from build123d import *

# Parameters (mm, degrees)
BASE_EXT_DEPTH            = 30
BASE_EXT_DEPTH_BACK       = 25
ESQUISSE1_W               = 165
ESQUISSE1_H               = 165
ESQUISSE1_R               = 2
ESQUISSE2_W               = 165
ESQUISSE2_H               = 165
ESQUISSE2_R               = 5
BASE_BAS_DEPTH            = 5
ACCES_START               = -6
ESQUISSE4_R               = 30
ACCES_ROUES_DEPTH         = 16
ESQUISSE7_R               = 2
VIDE_SUPPORT_MOTEUR_DEPTH = 5
ESQUISSE9_R               = 5
VIS_MOTEUR_10MM_DEPTH     = 2
ESQUISSE10_R              = 2
VIS_PATIN_DEPTH           = 5
VIDE_CROIX_DEPTH          = 11
VIDE_GUIDAGE_REACH        = 123.846


with BuildPart() as part:
    # Esquisse1 → BASE EXT (new, two sides: drawn at the far end of the back side and taken through both)
    with BuildSketch(Plane(origin=(0, 0, 0), x_dir=(1, 0, 0), z_dir=(0, 1, 0)).offset(-BASE_EXT_DEPTH_BACK)):
        Rectangle(ESQUISSE1_W, ESQUISSE1_H)
        with Locations(Location((-76.5, -76.5, 0), (0, 0, 270))):
            Circle(ESQUISSE1_R, mode=Mode.SUBTRACT)
        with Locations(Location((-76.5, 0, 0), (0, 0, 270))):
            Circle(ESQUISSE1_R, mode=Mode.SUBTRACT)
        with Locations(Location((76.5, -76.5, 0), (0, 0, 270))):
            Circle(ESQUISSE1_R, mode=Mode.SUBTRACT)
        with BuildLine():
            ThreePointArc((77.5, -69.066965626), (71.196699141, -71.196699141), (69.066965626, -77.5))
            Line((69.066965626, -77.5), (-69.066965626, -77.5))
            ThreePointArc((-69.066965626, -77.5), (-71.196699141, -71.196699141), (-77.5, -69.066965626))
            Line((-77.5, -69.066965626), (-77.5, -7.433034374))
            ThreePointArc((-77.5, -7.433034374), (-72.588712088, -6.399361443), (-69.428932188, -2.5))
            Line((-69.428932188, -2.5), (-7.071067812, -2.5))
            ThreePointArc((-7.071067812, -2.5), (0, -7.5), (7.071067812, -2.5))
            Line((7.071067812, -2.5), (69.428932188, -2.5))
            ThreePointArc((69.428932188, -2.5), (72.588712088, -6.399361443), (77.5, -7.433034374))
            Line((77.5, -7.433034374), (77.5, -69.066965626))
        make_face(mode=Mode.SUBTRACT)
        with Locations(Location((76.5, 0, 0), (0, 0, 270))):
            Circle(ESQUISSE1_R, mode=Mode.SUBTRACT)
        with BuildLine():
            Line((-7.071067812, 2.5), (-69.428932188, 2.5))
            ThreePointArc((-69.428932188, 2.5), (-72.588712088, 6.399361443), (-77.5, 7.433034374))
            Line((-77.5, 7.433034374), (-77.5, 69.066965626))
            ThreePointArc((-77.5, 69.066965626), (-71.196699141, 71.196699141), (-69.066965626, 77.5))
            Line((-69.066965626, 77.5), (-2, 77.5))
            Line((-2, 77.5), (-2, 7.228416147))
            ThreePointArc((-2, 7.228416147), (-5.114738276, 5.485385344), (-7.071067812, 2.5))
        make_face(mode=Mode.SUBTRACT)
        with Locations(Location((-76.5, 76.5, 0), (0, 0, 270))):
            Circle(ESQUISSE1_R, mode=Mode.SUBTRACT)
        with Locations(Location((0, 0, 0), (0, 0, 270))):
            Circle(ESQUISSE1_R, mode=Mode.SUBTRACT)
        with BuildLine():
            ThreePointArc((77.5, 7.433034374), (72.709235004, 6.471483659), (69.52750715, 2.76303157))
            Line((69.52750715, 2.76303157), (7.071067812, 2.5))
            ThreePointArc((7.071067812, 2.5), (5.114738276, 5.485385344), (2, 7.228416147))
            Line((2, 7.228416147), (2, 77.5))
            Line((2, 77.5), (69.066965626, 77.5))
            ThreePointArc((69.066965626, 77.5), (71.196699141, 71.196699141), (77.5, 69.066965626))
            Line((77.5, 69.066965626), (77.5, 7.433034374))
        make_face(mode=Mode.SUBTRACT)
        with Locations(Location((76.5, 76.5, 0), (0, 0, 270))):
            Circle(ESQUISSE1_R, mode=Mode.SUBTRACT)
    extrude(amount=BASE_EXT_DEPTH + BASE_EXT_DEPTH_BACK)

    # Esquisse2 → BASE BAS (add)
    with BuildSketch(Plane.XZ.offset(25)):
        Rectangle(ESQUISSE2_W, ESQUISSE2_H)
        with Locations(Location((-76.5, 0, 0), (0, 0, 270))):
            Circle(ESQUISSE2_R, mode=Mode.SUBTRACT)
        with Locations(Location((-76.5, -76.5, 0), (0, 0, 270))):
            Circle(ESQUISSE2_R, mode=Mode.SUBTRACT)
        with Locations(Location((76.5, -76.5, 0), (0, 0, 90))):
            Circle(ESQUISSE2_R, mode=Mode.SUBTRACT)
        with Locations(Location((76.5, 0, 0), (0, 0, 90))):
            Circle(ESQUISSE2_R, mode=Mode.SUBTRACT)
        with Locations(Location((76.5, 76.5, 0), (0, 0, 90))):
            Circle(ESQUISSE2_R, mode=Mode.SUBTRACT)
        with Locations(Location((0, 0, 0), (0, 0, 270))):
            Circle(ESQUISSE2_R, mode=Mode.SUBTRACT)
        with Locations(Location((-76.5, 76.5, 0), (0, 0, 270))):
            Circle(ESQUISSE2_R, mode=Mode.SUBTRACT)
    extrude(amount=BASE_BAS_DEPTH)

    # Esquisse4 → ACCES ROUES (cut)
    with BuildSketch(Plane(origin=(-77.5, 0, 0), x_dir=(0, 0, -1), z_dir=(1, 0, 0)).offset(ACCES_START)):
        with Locations((-38.25, -5.128631201)):
            Circle(ESQUISSE4_R)
    acces_roues = extrude(amount=ACCES_ROUES_DEPTH, mode=Mode.SUBTRACT)

    # SYM ACCES ROUE: ACCES ROUES across plane
    add(acces_roues.mirror(Plane(origin=(0, 0, 0), x_dir=(0, 0, 1), z_dir=(1, 0, 0))), mode=Mode.SUBTRACT)

    # Esquisse7 → VIDE SUPPORT MOTEUR (cut)
    with BuildSketch(Plane(origin=(0, -25, 0), x_dir=(1, 0, 0), z_dir=(0, 1, 0))):
        with Locations(Location((54.232363064, -61.25, 0), (0, 0, 270))):
            Circle(ESQUISSE7_R)
        with Locations(Location((31.732363064, -60.75, 0), (0, 0, 270))):
            Circle(ESQUISSE7_R)
        with Locations(Location((31.732363064, -15.75, 0), (0, 0, 270))):
            Circle(ESQUISSE7_R)
        with Locations(Location((54.232363064, -15.25, 0), (0, 0, 270))):
            Circle(ESQUISSE7_R)
        with Locations(Location((-54.232363064, -15.25, 0), (0, 0, 270))):
            Circle(ESQUISSE7_R)
        with Locations(Location((-31.732363064, -15.75, 0), (0, 0, 270))):
            Circle(ESQUISSE7_R)
        with Locations(Location((-31.732363064, -60.75, 0), (0, 0, 270))):
            Circle(ESQUISSE7_R)
        with Locations(Location((-54.232363064, -61.25, 0), (0, 0, 270))):
            Circle(ESQUISSE7_R)
    extrude(amount=-VIDE_SUPPORT_MOTEUR_DEPTH, mode=Mode.SUBTRACT)

    # Esquisse9 → VIS MOTEUR 10mm (cut)
    with BuildSketch(Plane.XZ.offset(30)):
        with Locations(Location((-54.232363064, 61.25, 0), (0, 0, 270))):
            Circle(ESQUISSE9_R)
        with Locations(Location((-31.732363064, 60.75, 0), (0, 0, 270))):
            Circle(ESQUISSE9_R)
        with Locations(Location((-54.232363064, 15.25, 0), (0, 0, 270))):
            Circle(ESQUISSE9_R)
        with Locations(Location((-31.732363064, 15.75, 0), (0, 0, 270))):
            Circle(ESQUISSE9_R)
        with Locations(Location((31.732363064, 15.75, 0), (0, 0, 90))):
            Circle(ESQUISSE9_R)
        with Locations(Location((54.232363064, 15.25, 0), (0, 0, 90))):
            Circle(ESQUISSE9_R)
        with Locations(Location((31.732363064, 60.75, 0), (0, 0, 90))):
            Circle(ESQUISSE9_R)
        with Locations(Location((54.232363064, 61.25, 0), (0, 0, 90))):
            Circle(ESQUISSE9_R)
    extrude(amount=-VIS_MOTEUR_10MM_DEPTH, mode=Mode.SUBTRACT)

    # Esquisse10 → VIS PATIN (cut)
    with BuildSketch(Plane.XZ.offset(30)):
        with Locations(Location((-42.5, -52.5, 0), (0, 0, 270))):
            Circle(ESQUISSE10_R)
        with Locations(Location((42.5, -52.5, 0), (0, 0, 270))):
            Circle(ESQUISSE10_R)
    extrude(amount=-VIS_PATIN_DEPTH, mode=Mode.SUBTRACT)

    # Esquisse11 → VIDE CROIX (cut)
    with BuildSketch(Plane.XY.offset(2.5)):
        Polygon((-69.428932188, 27.333215955), (-41.273544688, 2.5), (-69.428932188, -22.333215955), align=None)
        Polygon((-66.4053875, 30), (-38.25, 5.166784045), (-10.0946125, 30), align=None)
        Polygon((-7.071067812, -22.333215955), (-7.071067812, 27.333215955), (-35.226455312, 2.5), align=None)
        Polygon((-10.0946125, -25), (-66.4053875, -25), (-38.25, -0.166784045), align=None)
        Polygon((66.4053875, -25), (38.25, -0.166784045), (10.0946125, -25), align=None)
        Polygon((7.071067812, 27.333215955), (35.226455312, 2.5), (7.071067812, -22.333215955), align=None)
        Polygon((69.428932188, -22.333215955), (69.428932188, 27.333215955), (41.273544688, 2.5), align=None)
        Polygon((10.0946125, 30), (66.4053875, 30), (38.25, 5.166784045), align=None)
    extrude(amount=-VIDE_CROIX_DEPTH, mode=Mode.SUBTRACT)

    # VIDE GUIDAGE: up to this face of the body (flat: up to its plane)
    vide_guidage_end = Plane(part.part.faces().sort_by_distance((2, 2.5, -42.364208074))[0])
    # Esquisse12 → VIDE GUIDAGE (cut, up to the picked face)
    with BuildSketch(Plane.ZY.offset(2), mode=Mode.PRIVATE) as vide_guidage_sk1:
        Polygon((-7.228416147, 10), (-12.228416147, 10), (-12.228416147, 30), (-72.5, 30), (-72.5, 10), (-77.5, 10), (-77.5, -25), (-7.228416147, -25), align=None)
    vide_guidage_tool1 = split(extrude(vide_guidage_sk1.sketch, amount=-VIDE_GUIDAGE_REACH, mode=Mode.PRIVATE), bisect_by=vide_guidage_end, keep=Keep.BOTH, mode=Mode.PRIVATE)
    add(vide_guidage_tool1.solids().sort_by(Axis((-2, 1.545004, -42.364208), (1, 0, 0)))[0], mode=Mode.SUBTRACT)


solid = part.part
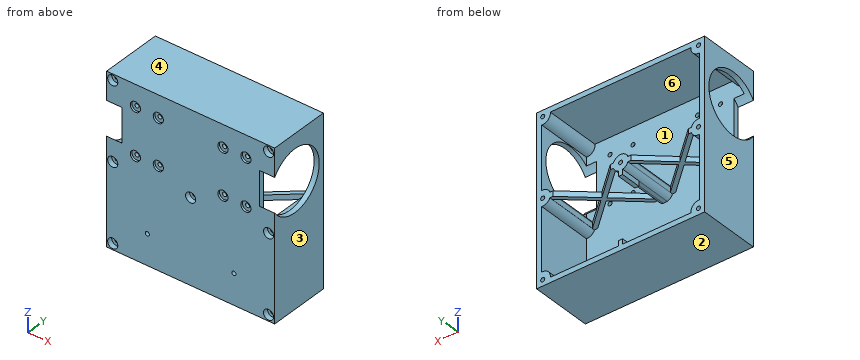
Input: part model. Units: mm. Frame: model coordinates. Face numbers are marked on the shaded views. A direction names the side the tool comes from. Give positions to 0.01 mm unless a question says otherwise; leave off trailing zeros. Order: outer loops, then holes, each group sorted by start corner. A loop starts at its lowest first (then second) coordinate and runs counter-clockwise, first axis right, second up. Notation, with made-up numbers: M 63.25,48.25 L 99.25,48.25 A3 ccw 99.25,53.25 Z; hole C 52,51 d1. An arc over 180 degrees is marked long. Answer as a JSON object with one key per item and string values.
1. Reachability of the marked faces 5 and 6 from +Z, -Z, +X, -X, +Y, -Y: full face, straight path, thin tool, end or side. Return the list, or none.
Result sheet:
{"face 5": "+Z, -Z, -X, +Y, -Y", "face 6": "+Y"}
2. Cut plane A-A, the plane z = 0. State how many separate pieces and enclosed holes the cut face has, and give its area (3 significant figures).
Result sheet:
{"separate pieces": "4", "enclosed holes": "6", "area": "3,500 mm²"}
3. Cut plane C-C, the plane z = -26. Output: boundary loops of the cut face in (x, y), and give its area (4 significant figures).
Result sheet:
{"outline": "M -82.5,-30 L 82.5,-30 L 82.5,30 L 77.5,30 L 77.5,-25 L -77.5,-25 L -77.5,30 L -82.5,30 Z", "area": "1,375 mm²"}
4. Cut plane B-B, the plane x = -24.5. Output: boundary loops of the cut face in (y, z).
Result sheet:
{"outline": "M -30,-82.5 L 30,-82.5 L 30,-77.5 L -25,-77.5 L -25,77.5 L 30,77.5 L 30,82.5 L -30,82.5 Z; M -12.29,-2.5 L -6.96,-2.5 L -6.96,2.5 L -12.29,2.5 Z; M 11.96,-2.5 L 17.29,-2.5 L 17.29,2.5 L 11.96,2.5 Z"}
5. Pull-direction query (Z, two-part tool) for the marked faces 1, 2, 3 and 4; classes: +Z half, -Z half, draft (parallel to the pull), parting line (faces both ways), or undercut.
Result sheet:
{"face 1": "undercut", "face 2": "-Z half", "face 3": "draft", "face 4": "+Z half"}
6. Cut plane D-D, the plane z = 41. Output: boundary loops of the cut face in (x, y).
Result sheet:
{"outline": "M -82.5,24.75 L -77.5,24.75 L -77.5,30 L -82.5,30 Z; M -67.5,-30 L 67.5,-30 L 67.5,-25 L -67.5,-25 Z; M 77.5,24.75 L 82.5,24.75 L 82.5,30 L 77.5,30 Z"}
7. First-contact query: P1, Ø1, axis at x = 38.5, z = 29, coming from the +Y side; P2, Ø5.5, axis at y = -28.5, z = 43, coming from the +X side; P3, Ø4.5, axis at x = -76.5, z = 0, coming from the -Y side. Flat tips, straight axial feed; report the tip coordinate or a pass-through.
Result sheet:
{"P1": "y = -25", "P2": "x = 67.5", "P3": "y = -25"}
8. Ray query, line 1 (X direction, y = -28.5, z = 60.75); line 2 (Z direction, x = 33, y = 9.5); line 3 (X direction, y = -26.3, z = 76.5). Return the intervals inside material, ascending. Write a range as [from, to].
Result sheet:
{"line 1": "[-82.5, -59.21], [-49.26, -36.73], [-26.73, 26.73], [36.73, 49.26], [59.21, 82.5]", "line 2": "[-82.5, -77.5], [-2.61, 2.5], [77.5, 82.5]", "line 3": "[-82.5, -81.5], [-71.5, 71.5], [81.5, 82.5]"}
